Check sheet for the modelled part. Datum: model origin and axes. Units: mm. A direction names the side the tool comes from. Give positions to 0.01 mm unless a question says otherwise; leave off trailing zeros. Order: outer loops, then holes, each group sorted by start corner. A loop starts at its lowest first (then second) coordinate and runs counter-clockwise, first axis right, second up. Notation, with made-up numbers: (7, 55.25) - (59, 55.25) arc R20 ccw to (59, 60.25) - close; hole circle Ø10 at (41, -36). An arc over 180 degrees is marked (long way). Answer in a Markdown table with one row per item.
from build123d import *

# Parameters (mm, degrees)
F0_R     = 11.049
F1_DEPTH = 25.4
F2_DEPTH = 50.8


# Not quite as in the source:
# - a feature names something its author has since deleted; it is built from what else it names


with BuildPart() as f1:
    # F0 (on Front) → F1 (new body)
    with BuildSketch(Plane.XZ):
        with BuildLine():
            ThreePointArc((101.6, 0), (94.1605122421, 17.9605122421), (76.2, 25.4))
            ThreePointArc((76.2, 25.4), (50.8, 0), (76.2, -25.4))
            ThreePointArc((76.2, -25.4), (94.1605122421, -17.9605122421), (101.6, 0))
        make_face()
        with Locations((76.2, 0)):
            Circle(F0_R, mode=Mode.SUBTRACT)
        with BuildLine():
            ThreePointArc((19.05, 25.4), (28.3980633142, 14.1990316571), (31.75, 0))
            ThreePointArc((31.75, 0), (28.3980633142, -14.1990316571), (19.05, -25.4))
            Line((19.05, -25.4), (76.2, -25.4))
            ThreePointArc((76.2, -25.4), (50.8, 0), (76.2, 25.4))
            Line((76.2, 25.4), (19.05, 25.4))
        make_face()
    extrude(amount=F1_DEPTH)

    # F0 (on Front) → F2 (join)
    with BuildSketch(Plane.XZ):
        with BuildLine():
            ThreePointArc((19.05, -25.4), (28.3980633142, -14.1990316571), (31.75, 0))
            ThreePointArc((31.75, 0), (28.3980633142, 14.1990316571), (19.05, 25.4))
            ThreePointArc((19.05, 25.4), (-31.75, 0), (19.05, -25.4))
        make_face()
        with BuildLine():
            ThreePointArc((15.1236685034, -4.826), (-15.875, 0), (15.1236685034, 4.826))
            Line((15.1236685034, 4.826), (19.9496685034, 4.826))
            Line((19.9496685034, 4.826), (19.9496685034, -4.826))
            Line((19.9496685034, -4.826), (15.1236685034, -4.826))
        make_face(mode=Mode.SUBTRACT)
    extrude(amount=F2_DEPTH)


solid = f1.part
(1) Cross-section at B-B, the plane y = -29.5. Record the cut outline in (x, z) (3 decimals), then the cut area to 3 significant figures.
Geometry says:
| item | result |
|---|---|
| outline | circle Ø63.5 at (0, 0); hole (15.124, -4.826) - (19.95, -4.826) - (19.95, 4.826) - (15.124, 4.826) arc R15.875 ccw (long way) to start |
| area | 2,330 mm² |
(2) Cross-section at D-D, the plane z = 18.5. Record the cut outline in (x, y).
Geometry says:
| item | result |
|---|---|
| outline | (-25.8, -50.8) - (25.8, -50.8) - (25.8, -25.4) - (93.6, -25.4) - (93.6, 0) - (-25.8, 0) - close |
(3) Thickness scan on L1, parallel to Z at x = 0, y = -26 (3 decimals); L2, parallel to Z at x = 76.2, y = -9.25; L3, parallel to X at y = -7, z = -9.5. Record the ranges inside material, lowest first.
Geometry says:
| item | result |
|---|---|
| L1 | -31.75 to -15.875, 15.875 to 31.75 |
| L2 | -25.4 to -11.05, 11.05 to 25.4 |
| L3 | -30.3 to -12.72, 12.72 to 70.56, 81.84 to 99.76 |
(4) Gauge pin test, flat ends, axial feed: P1, Ø2, axis at x = 51.5, z = -21, coming from the +Y side; P2, Ø5, axis at x = 38.5, y = -15, coming from the -Z side; P3, Ø15, axis at x = 66.5, z = 3, coming from the -Y side; P4, Ø3, axis at y = -43, z = -22, coming from the +X side. Record the tip position at first contact, or that the pin passes through.
Geometry says:
| item | result |
|---|---|
| P1 | y = 0 |
| P2 | z = -25.4 |
| P3 | y = -25.4 |
| P4 | x = 24.24 |
(5) Cross-section at C-C, the plane y = -12.5. Record the cut outline in (x, z) (3 decimals).
Geometry says:
| item | result |
|---|---|
| outline | (19.05, -25.4) - (76.2, -25.4) arc R25.4 ccw to (76.2, 25.4) - (19.05, 25.4) arc R31.75 ccw (long way) to start; hole (15.124, -4.826) - (19.95, -4.826) - (19.95, 4.826) - (15.124, 4.826) arc R15.875 ccw (long way) to start; hole circle Ø22.098 at (76.2, 0) |
(6) Cross-section at A-A, the plane x = 0. Record the cut outline in (y, z) (3 decimals), then the cut area to 3 significant figures.
Geometry says:
| item | result |
|---|---|
| outline | (-50.8, -31.75) - (0, -31.75) - (0, -15.875) - (-50.8, -15.875) - close; (-50.8, 15.875) - (0, 15.875) - (0, 31.75) - (-50.8, 31.75) - close |
| area | 1,610 mm² |
(7) Access from +Z, -Z, +X, -X, +Y, -Y to the whole of each face (thin tool, end or side, straight path). Record for faces 4 (the flat face through (18, -25, -4.826)), 5 (the flat face through (47, -13, -25.4)), 6 (the flat face through (34, 0, 0)).
Geometry says:
| item | result |
|---|---|
| face 4 | +Y, -Y |
| face 5 | -Z, +X, +Y, -Y |
| face 6 | +Z, -Z, +X, -X, +Y |
(8) Mould release check, pull along Z, two halves, no side actions. Record for faces 1 (the flat face through (60, -25.4, 0)), 2 (the cylindrical face through (-15.863, -25.044, -0.629)), 3 (the flat face through (48, -13, 25.4)): pulls with the +Z half, pulls with the -Z half, needs draft (parallel to the pull), parting line crosses it, or undercut.
Geometry says:
| item | result |
|---|---|
| face 1 | needs draft |
| face 2 | undercut |
| face 3 | pulls with the +Z half |
